Here's how the part is built. I have some questions about the finished solid (model axes, mm). Round coordinates to 2 decimals unless told otherwise and drop trailing zeros. Order: outer loops, then holes, each group sorted by start corner. A loop starts at its lowest first (then second) coordinate and runs counter-clockwise, first axis right, second up. Notation, with made-up numbers: (62.25, 76.25) -> (92.25, 76.25) arc R33 ccw to (92.25, 109.25) -> close; hole circle Ø9 at (20, -10.5). An arc over 180 degrees is marked (long way). Answer in a Markdown table with one row per item.
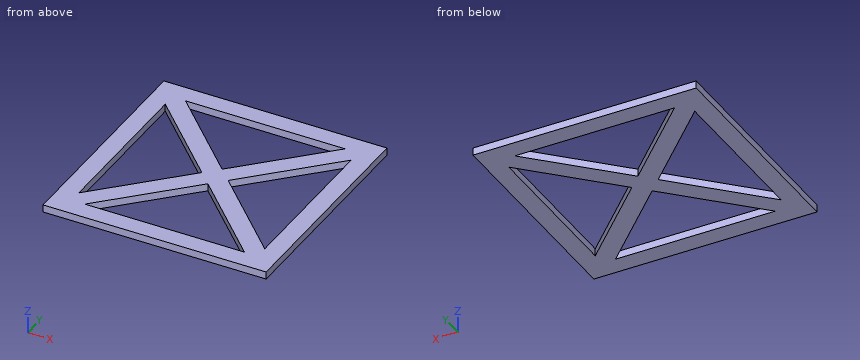
```python
from build123d import *

# Parameters (mm, degrees)
SKETCH1_W           = 300
SKETCH1_H           = 300
BOSS_EXTRUDE1_DEPTH = 10


with BuildPart() as part:
    # Sketch1 → Boss-Extrude1 (new body)
    with BuildSketch(Plane.XY):
        Rectangle(SKETCH1_W, SKETCH1_H)
        Polygon((-107.32233047, 125), (107.32233047, 125), (0, 17.67766953), align=None, mode=Mode.SUBTRACT)
        Polygon((125, -107.32233047), (125, 107.32233047), (17.67766953, 0), align=None, mode=Mode.SUBTRACT)
        Polygon((-107.32233047, -125), (107.32233047, -125), (0, -17.67766953), align=None, mode=Mode.SUBTRACT)
        Polygon((-125, -107.32233047), (-125, 107.32233047), (-17.67766953, 0), align=None, mode=Mode.SUBTRACT)
    extrude(amount=BOSS_EXTRUDE1_DEPTH)


solid = part.part
```
1. Please list where these lines run through material, in increasing order: line 1 along Y through (x, z) = (85.5, 7.75); line 2 along X through (y, z) = (63, 7); line 3 along Y through (x, z) = (-85, 3.5).
Numbers:
| item | result |
|---|---|
| line 1 | y = -150 to -125, -103.18 to -67.82, 67.82 to 103.18, 125 to 150 |
| line 2 | x = -150 to -125, -80.68 to -45.32, 45.32 to 80.68, 125 to 150 |
| line 3 | y = -150 to -125, -102.68 to -67.32, 67.32 to 102.68, 125 to 150 |
2. Suppose I cut it at B-B on y = -52.5. Write out the boundary of the cut face in (x, z).
Numbers:
| item | result |
|---|---|
| outline | (-150, 0) -> (-125, 0) -> (-125, 10) -> (-150, 10) -> close; (-70.18, 0) -> (-34.82, 0) -> (-34.82, 10) -> (-70.18, 10) -> close; (34.82, 0) -> (70.18, 0) -> (70.18, 10) -> (34.82, 10) -> close; (125, 0) -> (150, 0) -> (150, 10) -> (125, 10) -> close |
3. Suppose I cut it at A-A on z = 6.5. Write out the boundary of the cut face in (x, y).
Numbers:
| item | result |
|---|---|
| outline | (-150, -150) -> (150, -150) -> (150, 150) -> (-150, 150) -> close; hole (-125, -107.32) -> (-17.68, 0) -> (-125, 107.32) -> close; hole (-107.32, -125) -> (107.32, -125) -> (0, -17.68) -> close; hole (-107.32, 125) -> (0, 17.68) -> (107.32, 125) -> close; hole (17.68, 0) -> (125, -107.32) -> (125, 107.32) -> close |
4. Suppose I cut it at C-C on x = -56.5. Write out the boundary of the cut face in (y, z), then the cut area to 3 significant figures.
Numbers:
| item | result |
|---|---|
| outline | (-150, 0) -> (-125, 0) -> (-125, 10) -> (-150, 10) -> close; (-74.18, 0) -> (-38.82, 0) -> (-38.82, 10) -> (-74.18, 10) -> close; (38.82, 0) -> (74.18, 0) -> (74.18, 10) -> (38.82, 10) -> close; (125, 0) -> (150, 0) -> (150, 10) -> (125, 10) -> close |
| area | 1,210 mm2 |
5. Suppose I cut it at D-D on y = 115. Write out the boundary of the cut face in (x, z).
Numbers:
| item | result |
|---|---|
| outline | (-150, 0) -> (-97.32, 0) -> (-97.32, 10) -> (-150, 10) -> close; (97.32, 0) -> (150, 0) -> (150, 10) -> (97.32, 10) -> close |
